Geometry: final body of the model. Coordinates: model frame, mm. A direction names the side the tool comes from. Coordinates: 2 decimals unless noted, no trailing zeros. Order: outer loops, then holes, each group sorted by start corner. A loop starts at its lowest first (then second) coordinate and runs counter-clockwise, first axis right, second up. Notation, with made-up numbers: (89, 71.25) - (119, 71.25) arc R31 ccw to (119, 109.25) - close; hole circle Ø6 at (4.5, 83.25). An arc over 180 degrees is marked (long way). Use a Markdown table: item, result. Add a question column.
```python
from build123d import *

# Parameters (mm, degrees)
SKETCH_1_W          = 250
SKETCH_1_H          = 20
SKETCH_1_R          = 3.25
EXTRUDE_1_DEPTH     = 5
SKETCH_2_R          = 5.6
CUT_EXTRUDE_1_DEPTH = 2.5
CUT_EXTRUDE_START   = -2.5
SKETCH_3_R          = 5.6
CUT_EXTRUDE_2_DEPTH = 2.5
SKETCH_4_R          = 2.1
CUT_EXTRUDE_3_DEPTH = 126.797456254
FILLET_1_R          = 2


with BuildPart() as part:
    # 草图1 → 凸台-拉伸1 (new, symmetric)
    with BuildSketch(Plane.XY):
        Rectangle(SKETCH_1_W, SKETCH_1_H)
        Circle(SKETCH_1_R, mode=Mode.SUBTRACT)
    extrude(amount=EXTRUDE_1_DEPTH, both=True)

    # 草图2 → 切除-拉伸1 (cut)
    with BuildSketch(Plane(origin=(0, 0, -5), x_dir=(-1, 0, 0), z_dir=(0, 0, -1))):
        Circle(SKETCH_2_R)
    extrude(amount=-CUT_EXTRUDE_1_DEPTH, mode=Mode.SUBTRACT)

    # 草图3 → 切除-拉伸2 (cut)
    with BuildSketch(Plane.XY.offset(5).offset(CUT_EXTRUDE_START)):
        with Locations(Location((0, 0, 0), (0, 0, 180))):
            Circle(SKETCH_3_R)
    extrude(amount=CUT_EXTRUDE_2_DEPTH, mode=Mode.SUBTRACT)

    # 草图4 → 切除-拉伸3 (cut, through all)
    with BuildSketch(Plane.XY.offset(5)):
        with Locations((-120, 5)):
            Circle(SKETCH_4_R)
        with Locations((-120, -5)):
            Circle(SKETCH_4_R)
        with Locations(Location((120, -5, 0), (0, 0, 180))):
            Circle(SKETCH_4_R)
        with Locations(Location((120, 5, 0), (0, 0, 180))):
            Circle(SKETCH_4_R)
    extrude(amount=-CUT_EXTRUDE_3_DEPTH, mode=Mode.SUBTRACT)

    # 圆角1
    fillet_1_edges = [part.edges().sort_by_distance(p)[0] for p in [
        (0, -10, 5),
        (0, -10, -5),
        (0, 10, -5),
        (0, 10, 5),
    ]]
    fillet(fillet_1_edges, radius=FILLET_1_R)


solid = part.part
```
1) Section query A-A (x = -120). Return the cut outline in (y, z).
2) Draft query along Y for faces 1 (the cylindrical face through (118.06, 5.8, 0.07)), 2 (the flat face through (-125, 0, 0)), 3 (the flat face through (-2.41, -2.41, -2.5)), 4 (the flat face through (-2, -10, 0)). Return one class per face: released by +Y, released by -Y, zero draft, split by the parting line, or undercut.
3) Section query C-C (z = -0.5). Return the cut outline in (x, y).
4) Section query D-D (x = 0). Return the cut outline in (y, z), and give its area (3 significant figures).
5) First-contact query: pin 1 (3.5 mm diameter, centred on x = -120, y = -5, fed in from -Z); pin 2 (7.5 mm diameter, centred on x = 0, y = 0, fed in from -Z). Flat tips, straight axial feed; report the tip coordinate or a pass-through.
6) Access query for faces 5 (the flat face through (-2, 7, 5)), 6 (the flat face through (-2.41, 2.41, 2.5)), 7 (the cylindrical face through (5.595, 0.246, -3.768)). Directions: +Z, -Z, +X, -X, +Y, -Y. A direction counts if a zero-diameter tool reaches every point of the face in a straight line with its end or side. Return the directions, or none.
7) Section query B-B (y = 0). Return the cut outline in (x, z), and give its area (3 significant figures).
8) Line query: line 1 (Y direction, x = 120, z = 1); line 2 (X direction, y = 0, z = 1.05); line 3 (Z direction, x = 102.5, y = 8.25). Output: solid intervals per line, ascending. Write a range as from..to.
From the geometry:
| question | item | result |
|---|---|---|
| 1 | outline | (-10, -3) arc R2 ccw to (-8, -5) - (-7.1, -5) - (-7.1, 5) - (-8, 5) arc R2 ccw to (-10, 3) - close; (-2.9, -5) - (2.9, -5) - (2.9, 5) - (-2.9, 5) - close; (7.1, -5) - (8, -5) arc R2 ccw to (10, -3) - (10, 3) arc R2 ccw to (8, 5) - (7.1, 5) - close |
| 2 | face 1 | undercut |
| 2 | face 2 | zero draft |
| 2 | face 3 | undercut |
| 2 | face 4 | released by -Y |
| 3 | outline | (-125, -10) - (125, -10) - (125, 10) - (-125, 10) - close; hole circle Ø4.2 at (-120, -5); hole circle Ø4.2 at (-120, 5); hole circle Ø6.5 at (0, 0); hole circle Ø4.2 at (120, -5); hole circle Ø4.2 at (120, 5) |
| 4 | outline | (-10, -3) arc R2 ccw to (-8, -5) - (-5.6, -5) - (-5.6, -2.5) - (-3.25, -2.5) - (-3.25, 2.5) - (-5.6, 2.5) - (-5.6, 5) - (-8, 5) arc R2 ccw to (-10, 3) - close; (3.25, -2.5) - (5.6, -2.5) - (5.6, -5) - (8, -5) arc R2 ccw to (10, -3) - (10, 3) arc R2 ccw to (8, 5) - (5.6, 5) - (5.6, 2.5) - (3.25, 2.5) - close |
| 4 | area | 108 mm^2 |
| 5 | pin 1 | passes through |
| 5 | pin 2 | stops at z = -2.5 |
| 6 | face 5 | +Z, +X, -X, +Y, -Y |
| 6 | face 6 | +Z |
| 6 | face 7 | -Z |
| 7 | outline | (-125, -5) - (-5.6, -5) - (-5.6, -2.5) - (-3.25, -2.5) - (-3.25, 2.5) - (-5.6, 2.5) - (-5.6, 5) - (-125, 5) - close; (3.25, -2.5) - (5.6, -2.5) - (5.6, -5) - (125, -5) - (125, 5) - (5.6, 5) - (5.6, 2.5) - (3.25, 2.5) - close |
| 7 | area | 2,410 mm^2 |
| 8 | line 1 | y = -10..-7.1, -2.9..2.9, 7.1..10 |
| 8 | line 2 | x = -125..-3.25, 3.25..125 |
| 8 | line 3 | z = -4.98..4.98 |
